Could you check a few things on this model? Use its own coordinates, in mm. A direction names the side the tool comes from. Give positions to 0.01 mm unless a question says otherwise; leave off trailing zeros. Order: outer loops, then holes, each group sorted by start corner. A loop starts at its lowest first (then second) coordinate and runs counter-clockwise, first axis right, second up. Notation, with made-up numbers: (7.25, 7) -> (56.25, 7) arc R16 cw to (56.25, 28) -> close; hole circle Ø7 at (53, 82.25). An arc over 180 degrees is marked (long way). Write each question's results on one line, items separated by ' | '.
```python
from build123d import *

# Parameters (mm, degrees)
SKETCH1_R           = 2.25
BOSS_EXTRUDE1_DEPTH = 25.4
FILLET2_R           = 5
SKETCH3_R           = 2.25
CUT_EXTRUDE2_DEPTH  = 178.913356722
FILLET4_R           = 12.7
FILLET6_R           = 6.35
FILLET5_R           = 1


with BuildPart() as part:
    # Sketch1 → Boss-Extrude1 (new body)
    with BuildSketch(Plane(origin=(0, 0, 0), x_dir=(1, 0, 0), z_dir=(0, 1, 0))):
        Polygon((53.761053629, 31.75), (75.074184261, 57.15), (158.75, 57.15), (158.75, 69.85), (69.152077003, 69.85), (47.838946371, 44.45), (13.874173221, 44.45), (-6.35, 27.479903709), (-6.35, -6.35), (6.35, -6.35), (6.35, 23.320096291), (16.39636803, 31.75), align=None)
        with Locations(Location((0, 0, 0), (0, 0, 270))):
            Circle(SKETCH1_R, mode=Mode.SUBTRACT)
        with Locations(Location((0, 12.7, 0), (0, 0, 270))):
            Circle(SKETCH1_R, mode=Mode.SUBTRACT)
        with Locations(Location((0, 25.4, 0), (0, 0, 270))):
            Circle(SKETCH1_R, mode=Mode.SUBTRACT)
        with Locations(Location((152.4, 63.5, 0), (0, 0, 270))):
            Circle(SKETCH1_R, mode=Mode.SUBTRACT)
        with Locations(Location((139.7, 63.5, 0), (0, 0, 270))):
            Circle(SKETCH1_R, mode=Mode.SUBTRACT)
    extrude(amount=BOSS_EXTRUDE1_DEPTH)

    # Fillet2
    fillet2_edges = [part.edges().sort_by_distance(p)[0] for p in [
        (6.35, 12.7, 6.35),
        (-6.35, 12.7, 6.35),
    ]]
    fillet(fillet2_edges, radius=FILLET2_R)

    # Sketch3 → Cut-Extrude2 (cut, through all)
    with BuildSketch(Plane(origin=(0, 0, -69.85), x_dir=(-1, 0, 0), z_dir=(0, 0, -1))):
        with Locations((-31.75, 6.35)):
            Circle(SKETCH3_R)
        with Locations((-31.75, 19.05)):
            Circle(SKETCH3_R)
        with Locations(Location((-139.7, 12.7, 0), (0, 0, 180))):
            Circle(SKETCH3_R)
    extrude(amount=-CUT_EXTRUDE2_DEPTH, mode=Mode.SUBTRACT)

    # Fillet4
    fillet4_edges = [part.edges().sort_by_distance(p)[0] for p in [
        (-6.35, 12.7, -27.479903709),
        (13.874173221, 12.7, -44.45),
        (47.838946371, 12.7, -44.45),
        (69.152077003, 12.7, -69.85),
        (75.074184261, 12.7, -57.15),
        (53.761053629, 12.7, -31.75),
        (16.39636803, 12.7, -31.75),
        (6.35, 12.7, -23.320096291),
    ]]
    fillet(fillet4_edges, radius=FILLET4_R)

    # Fillet6
    fillet6_edges = [part.edges().sort_by_distance(p)[0] for p in [
        (158.75, 12.7, -69.85),
        (158.75, 12.7, -57.15),
    ]]
    fillet(fillet6_edges, radius=FILLET6_R - 0.0001)  # a hair under: the kernel refuses the full size

    # Fillet5
    fillet5_edges = [part.edges().sort_by_distance(p)[0] for p in [
        (113.737142131, 25.4, -69.85),
        (6.35, 25.4, -8.023994516),
        (11.87099236, 25.4, -27.952758944),
        (34.428868188, 25.4, -31.75),
        (64.417618945, 25.4, -44.45),
        (30.206717154, 25.4, -44.45),
        (4.259894955, 25.4, -36.382662653),
        (-5.160108895, 25.4, -26.925048375),
        (14.152939376, 25.4, -43.684096284),
        (53.206198295, 25.4, -32.939891105),
        (69.706932337, 25.4, -68.660108895),
        (47.284091036, 0, -45.639891105),
        (47.284091036, 25.4, -45.639891105),
        (75.629039596, 0, -55.960108895),
        (75.629039596, 25.4, -55.960108895),
        (16.675134185, 0, -30.984096284),
        (16.675134185, 25.4, -30.984096284),
        (7.539891105, 0, -22.765240957),
        (7.539891105, 25.4, -22.765240957),
        (116.69819576, 0, -57.15),
        (156.89015735, 0, -59.00984265),
        (156.89015735, 0, -67.99015735),
        (116.69819576, 25.4, -57.15),
        (156.89015735, 25.4, -59.00984265),
        (156.89015735, 25.4, -67.99015735),
        (0, 0, 6.35),
        (0, 25.4, 6.35),
        (-6.35, 0, -10.103898225),
        (4.885533906, 0, 4.885533906),
        (-4.885533906, 0, 4.885533906),
        (-6.35, 25.4, -10.103898225),
        (4.885533906, 25.4, 4.885533906),
        (-4.885533906, 25.4, 4.885533906),
        (58.495511687, 0, -57.15),
        (58.495511687, 25.4, -57.15),
        (4.259894955, 0, -36.382662653),
        (30.206717154, 0, -44.45),
        (113.737142131, 0, -69.85),
        (64.417618945, 0, -44.45),
        (34.428868188, 0, -31.75),
        (11.87099236, 0, -27.952758944),
        (6.35, 0, -8.023994516),
        (-5.160108895, 0, -26.925048375),
        (14.152939376, 0, -43.684096284),
        (53.206198295, 0, -32.939891105),
        (69.706932337, 0, -68.660108895),
    ]]
    fillet(fillet5_edges, radius=FILLET5_R)


solid = part.part
```
Q1. Suppose I cut it at B-B on x = 31.75. Please give me the cut outline in (y, z), and give its area (3 significant figures).
Here are the results:
outline: (0, -43.45) arc R1 ccw to (1, -44.45) -> (4.1, -44.45) -> (4.1, -31.75) -> (1, -31.75) arc R1 ccw to (0, -32.75) -> close; (8.6, -44.45) -> (16.8, -44.45) -> (16.8, -31.75) -> (8.6, -31.75) -> close; (21.3, -44.45) -> (24.4, -44.45) arc R1 ccw to (25.4, -43.45) -> (25.4, -32.75) arc R1 ccw to (24.4, -31.75) -> (21.3, -31.75) -> close | area: 207 mm²
Q2. I'm going to push flat-ended pins straight in: pin 1 Ø1.5 at (y, z) = (9, -52) entering from +X; pin 2 Ø7 at (x, z) = (152.4, -63.5) entering from +Y; pin 3 Ø10 at (y, z) = (16, -31.5) entering from +X; pin 4 Ø6 at (x, y) = (31.75, 19.05) entering from -Z. Where does each tip first touch, or does it pass through?
Here are the results:
pin 1: stops at x = 71.38 | pin 2: stops at y = 25.4 | pin 3: stops at x = 57.75 | pin 4: stops at z = -44.45
Q3. For faces 1 (the cylindrical face through (58.822, 0.285, -57.071)), 2 (the flat face through (30, 13, -44.45)), 3 (the flat face through (34, 13, -31.75)), which set-ups out of +Z, -Z, +X, -X, +Y, -Y let a thin tool reach every point of the face, with its end or its side?
Here are the results:
face 1: -Z, -X, -Y | face 2: -Z, -X, +Y, -Y | face 3: +Z, +X, +Y, -Y
Q4. Suppose I cut it at D-D on z = -6.5. Please give me the cut outline in (x, y).
Here are the results:
outline: (-6.35, 1) arc R1 ccw to (-5.35, 0) -> (5.35, 0) arc R1 ccw to (6.35, 1) -> (6.35, 24.4) arc R1 ccw to (5.35, 25.4) -> (-5.35, 25.4) arc R1 ccw to (-6.35, 24.4) -> close
Q5. I need wall thicknesses on line 1 along Y through (x, z) = (31.75, -42); line 2 along Z through (x, y) = (139.7, 6.5); line 3 along Y through (x, z) = (139.7, -68.25). Which ranges of each line are inside material? Lowest first, please.
Here are the results:
line 1: y = 0 to 4.1, 8.6 to 16.8, 21.3 to 25.4 | line 2: z = -69.85 to -65.75, -61.25 to -57.15 | line 3: y = 0 to 10.45, 14.95 to 25.4
Q6. Suppose I cut it at C-C on x = 139.7. Please give me the cut outline in (y, z), and give its area (3 significant figures).
Here are the results:
outline: (0, -68.85) arc R1 ccw to (1, -69.85) -> (10.45, -69.85) -> (10.45, -65.75) -> (0, -65.75) -> close; (0, -61.25) -> (10.45, -61.25) -> (10.45, -57.15) -> (1, -57.15) arc R1 ccw to (0, -58.15) -> close; (14.95, -69.85) -> (24.4, -69.85) arc R1 ccw to (25.4, -68.85) -> (25.4, -65.75) -> (14.95, -65.75) -> close; (14.95, -61.25) -> (25.4, -61.25) -> (25.4, -58.15) arc R1 ccw to (24.4, -57.15) -> (14.95, -57.15) -> close | area: 171 mm²
Q7. Suppose I cut it at A-A on y = 6.35. State how many separate pieces and enclosed holes the cut face has, and give its area (3 significant figures).
Here are the results:
separate pieces: 2 | enclosed holes: 5 | area: 2,440 mm²
Q8. Thinking about a two-plate mould opening in X: for faces 4 (the cylindrical face through (4.36, 25.1, -36.09)), 5 (the cylindrical face through (53.14, 12.86, -32.91)), 6 (the flat face through (116, 13, -57.15)), 7 (the cylindrical face through (0.676, 12.522, 2.146)), which applies, +X half, -X half, draft (parallel to the pull), parting line (faces both ways), or undercut?
Here are the results:
face 4: -X half | face 5: +X half | face 6: draft | face 7: undercut
